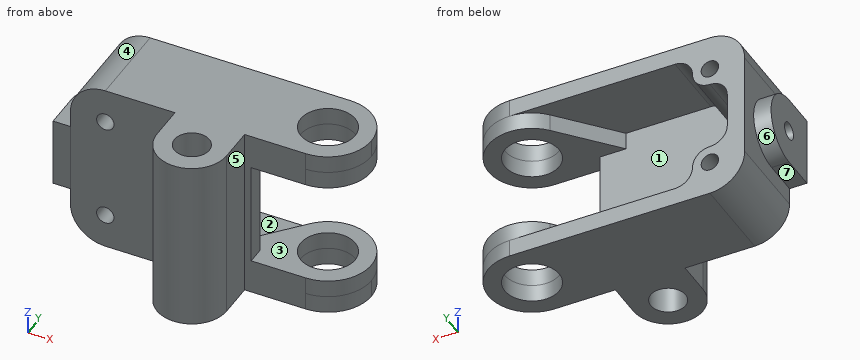
from build123d import *
from build123d.topology import SkipClean

# Parameters (mm, degrees)
SKETCH1_R           = 8
BOSS_EXTRUDE1_DEPTH = 40
SKETCH2_W           = 45
SKETCH2_H           = 64
CUT_EXTRUDE1_DEPTH  = 80
FILLET1_R           = 20
HOLE1_D             = 25
FILLET2_R           = 16
HOLE2_D             = 8
CUT_EXTRUDE2_DEPTH  = 32
SKETCH8_R           = 12.5
BOSS_EXTRUDE2_DEPTH = 8
BOSS_EXTRUDE3_DEPTH = 8
HOLE3_D             = 8


with BuildPart() as part:
    # Sketch1 → Boss-Extrude1 (new, symmetric)
    with BuildSketch(Plane.XY):
        with BuildLine():
            Line((48, -16), (48, 0))
            Line((48, 0), (0, 0))
            Line((0, 0), (0, 40))
            Line((0, 40), (128, 40))
            Line((128, 40), (128, 0))
            Line((128, 0), (80, 0))
            Line((80, 0), (80, -16))
            ThreePointArc((80, -16), (64, -32), (48, -16))
        make_face()
        with Locations((64, -16)):
            Circle(SKETCH1_R, mode=Mode.SUBTRACT)
    extrude(amount=BOSS_EXTRUDE1_DEPTH, both=True)

    # Sketch2 → Cut-Extrude1 (cut)
    with BuildSketch(Plane(origin=(0, 40, 0), x_dir=(1, 0, 0), z_dir=(0, 1, 0))):
        with Locations((105.5, 0)):
            Rectangle(SKETCH2_W, SKETCH2_H)
    extrude(amount=-CUT_EXTRUDE1_DEPTH, mode=Mode.SUBTRACT)

    # Fillet1
    fillet1_edges = [part.edges().sort_by_distance(p)[0] for p in [
        (128, 0, 36),
        (128, 0, -36),
        (128, 40, -36),
        (128, 40, 36),
    ]]
    fillet(fillet1_edges, radius=FILLET1_R - 0.0001)  # a hair under: the kernel refuses the full size

    # Hole1 (through all)
    with Locations(Plane.XY.offset(40)):
        with Locations((108, 20)):
            Hole(HOLE1_D / 2)

    # Fillet2
    fillet2_edges = [part.edges().sort_by_distance(p)[0] for p in [
        (0, 20, -40),
        (0, 20, 40),
    ]]
    fillet(fillet2_edges, radius=FILLET2_R)

    # Hole2 (through all)
    with Locations(Plane(origin=(0, 40, 0), x_dir=(1, 0, 0), z_dir=(0, 1, 0))):
        with Locations((16, 24), (16, -24)):
            Hole(HOLE2_D / 2)

    # Sketch7 → Cut-Extrude2 (cut)
    with BuildSketch(Plane(origin=(0, 40, 0), x_dir=(1, 0, 0), z_dir=(0, 1, 0))):
        with BuildLine():
            Line((8, -8), (8, 8))
            ThreePointArc((8, 8), (10.343145751, 13.656854249), (16, 16))
            ThreePointArc((16, 16), (21.656854249, 18.343145751), (24, 24))
            ThreePointArc((24, 24), (26.343145751, 29.656854249), (32, 32))
            Line((32, 32), (83, 32))
            Line((83, 32), (83, -32))
            Line((83, -32), (32, -32))
            ThreePointArc((32, -32), (26.343145751, -29.656854249), (24, -24))
            ThreePointArc((24, -24), (21.656854249, -18.343145751), (16, -16))
            ThreePointArc((16, -16), (10.343145751, -13.656854249), (8, -8))
        make_face()
    extrude(amount=-CUT_EXTRUDE2_DEPTH, mode=Mode.SUBTRACT)

    # Sketch8 → Boss-Extrude2 (add)
    with SkipClean():  # the faces are left unmerged after this step: merging them gives an invalid solid
        with BuildSketch(Plane.XY.offset(-32)):
            with BuildLine():
                Line((83, 8), (71, 8))
                Line((71, 8), (92.926108981, 33.14449731))
                ThreePointArc((92.926108981, 33.14449731), (126.205630258, 28.279796308), (108, 0))
                Line((108, 0), (83, 0))
                Line((83, 0), (83, 8))
            make_face()
            with Locations((108, 20)):
                Circle(SKETCH8_R, mode=Mode.SUBTRACT)
        boss_extrude2 = extrude(amount=BOSS_EXTRUDE2_DEPTH)
    add(part.part.scale(1), mode=Mode.REPLACE)  # the faces are merged on a copy

    # Mirror1: Boss-Extrude2 across plane
    add(boss_extrude2.mirror(Plane.XY))

    # Sketch9 → Boss-Extrude3 (add)
    with BuildSketch(Plane.ZY):
        with BuildLine():
            Line((-16, 16), (-16, 0))
            Line((-16, 0), (16, 0))
            Line((16, 0), (16, 16))
            ThreePointArc((16, 16), (0, 32), (-16, 16))
        make_face()
    extrude(amount=BOSS_EXTRUDE3_DEPTH)

    # Hole3 (through all)
    with Locations(Plane.ZY.offset(8)):
        with Locations((0, 16)):
            Hole(HOLE3_D / 2)


solid = part.part
The listing builds one solid part. Answer for the finished solid, in the listing's coordinates (mm). Face numbers are marked on the shaded views. A direction names the side the tool comes from. Coordinates: 2 decimals unless noted, no trailing zeros. Write each loop counter-clockwise with the first axis right and the second up, starting at its lowest first coordinate (ties: lowest second). Pieces come first, ordered by that corner, then holes. Notation, with made-up numbers: M 1.5,20.5 L 55.5,20.5 A15 ccw 55.5,48.5 Z; hole C 34.5,34 d1. An arc over 180 degrees is marked long. Put each result on its own line as item: value. Start each with the question number.
1. A cutting plane is placed at B-B on x = 57.5. Write down the section's boundary in (y, z).
2. A cutting plane is placed at A-A on z = 0. Write down the section's boundary in (x, y).
3. A cutting plane is placed at D-D on y = 35. Write down the section's boundary in (x, z).
4. Flat-ended cylindrical pins translate along their axes: P1, Ø12, axis at y = 22.5, z = -23, coming from the -X side; P2, Ø4, axis at y = 5, z = -4, coming from the +X side; P3, Ø5, axis at y = -6, z = -17, coming from the -X side. Find the tip coordinate at first contact, or state that the pin passes through.
5. Which of the six approach directions +Z, -Z, +X, -X, +Y, -Y give full straight-line access (tool end or side, diameter ignored) to the marked faces 5, 6 and 7?
6. A cutting plane is placed at C-C on x = 116. Count the separate pieces of the cut face and the enclosed holes in it, then the cut area to 3 significant figures.
7. Consider line 1 (Z direction, x = 16, y = 29); line 2 (Y direction, x = 108, z = -27); line 3 (Z direction, x = 84, y = 3.5). Determine where each line is inside the solid, lowest interval first. Write a range as from..to.
8. For a pull along X with two mould halves and no side action, classify the marked faces 1, 2, 3 and 4 as pulls with the +X half, pulls with the -X half, needs draft (parallel to the pull), parting line crosses it, or undercut.
Resolved:
1. outline: M -30.62,-40 L -20.66,-40 L -20.66,40 L -30.62,40 Z; M -11.34,-40 L 40,-40 L 40,-32 L 8,-32 L 8,32 L 40,32 L 40,40 L -11.34,40 Z
2. outline: M -8,0 L 48,0 L 48,-16 A16 ccw 80,-16 L 80,0 L 83,0 L 83,8 L 8,8 L 8,12 L -8,12 Z; M -8,20 L 8,20 L 8,40 L 0,40 L 0,32 L -8,32 Z; hole C 64,-16 d16
3. outline: M 0,-24 A16 ccw 16,-40 L 121.23,-40 L 121.23,-24 L 94.77,-24 L 94.77,-32 L 32,-32 A8 cw 24,-24 A8 ccw 16,-16 A8 cw 8,-8 L 8,8 A8 cw 16,16 A8 ccw 24,24 A8 cw 32,32 L 94.77,32 L 94.77,24 L 121.23,24 L 121.23,40 L 16,40 A16 ccw 0,24 Z; hole C 16,-24 d8; hole C 16,24 d8
4. P1: stops at x = 0
4. P2: stops at x = 83
4. P3: stops at x = 48
5. face 5: +Z, -Z, +X, -Y
5. face 6: -X, +Y
5. face 7: -Z, -X, +Y, -Y
6. separate pieces: 4
6. enclosed holes: 0
6. area: 558 mm2
7. line 1: z = -40..-28, -20..-16, 16..20, 28..40
7. line 2: y = 0..7.5, 32.5..40
7. line 3: z = -40..-24, 24..40
8. face 1: undercut
8. face 2: undercut
8. face 3: needs draft
8. face 4: pulls with the -X half
